Read the model definition and answer for the solid it produces. Units are mm, in the model's axes. Face numbers are marked on the shaded views. A direction names the side the tool comes from. Coordinates: 2 decimals unless noted, no trailing zeros. Write each loop counter-clockwise with the first axis right and the second up, starting at its lowest first coordinate (ties: lowest second). Pieces come first, ordered by that corner, then holes.
Item 1: A tool of negligible diameter and unlimited length cuts with its end or side. For the marked faces 1, 2, 3, 4 and 5, from which of +Z, -Z, +X, -X, +Y, -Y can it reach the whole face along a straight path? Write none if from no direction.
Item 2: This flat-tipped pin is pushed along its axis until it touches: P1, Ø3, axis at x = 24.5, y = 3, coming from the +Z side. Where does it stop, or does it pass through?
Item 3: Straight lines are drawn through the part: probe 1 along X at (y, z) = (1.2, -5); probe 2 along Z at (x, y) = (7, 4.35); probe 3 along X at (y, z) = (3.15, -24). For each, find the intervals that lie inside material, in ascending order.
Item 4: Section A-A (x = 43) is taken. Give the vertices of the cut face in (y, z).
Item 5: Determine the mould class of the marked faces 6, 7, 8 and 9 for opening direction Z: released by +Z, released by -Z, zero draft, split by the parting line, or undercut.
Item 6: Section C-C (x = 27) is taken. Give the vertices of the cut face in (y, z).
Item 7: Section B-B (y = 5.1) is taken. Give the vertices of the cut face in (x, z).
Item 8: Section D-D (z = -24) is taken. Give the vertices of the cut face in (x, y).
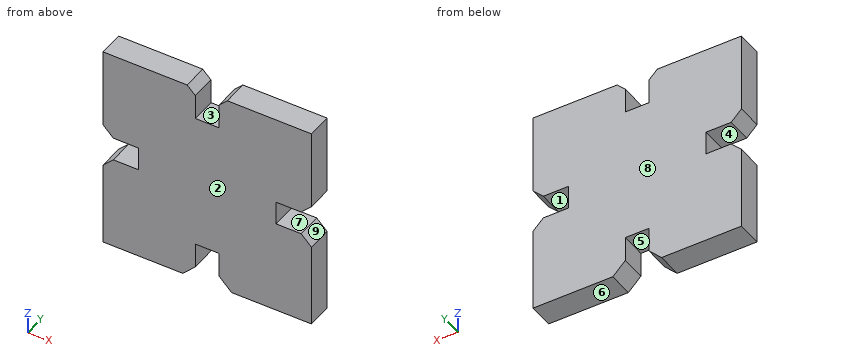
from build123d import *

# Parameters (mm, degrees)
SKETCH1_W           = 50
SKETCH1_H           = 50
BOSS_EXTRUDE1_DEPTH = 6
SKETCH2_W           = 5.7
SKETCH2_H           = 9
CUT_EXTRUDE1_DEPTH  = 6
CHAMFER2_SIZE       = 3
CIRPATTERN4_DEPTH   = 6


# Read off the part's stored shape, not the designer's step: CirPattern4
with BuildPart() as part:
    # Sketch1 → Boss-Extrude1 (new body)
    with BuildSketch(Plane(origin=(0, 0, 0), x_dir=(1, 0, 0), z_dir=(0, 1, 0))):
        with Locations((25, 25)):
            Rectangle(SKETCH1_W, SKETCH1_H)
    extrude(amount=BOSS_EXTRUDE1_DEPTH)

    # Sketch2 → Cut-Extrude1 (cut)
    with BuildSketch(Plane(origin=(0, 6, 0), x_dir=(1, 0, 0), z_dir=(0, 1, 0))):
        with Locations((25, 45.5)):
            Rectangle(SKETCH2_W, SKETCH2_H)
    extrude(amount=-CUT_EXTRUDE1_DEPTH, mode=Mode.SUBTRACT)

    # Chamfer2
    chamfer2_edges = [part.edges().sort_by_distance(p)[0] for p in [
        (22.15, 3, -50),
        (27.85, 3, -50),
    ]]
    chamfer(chamfer2_edges, length=CHAMFER2_SIZE)

    # CirPattern4 outline → CirPattern4 (cut)
    with BuildSketch(Plane(origin=(0, 0, 0), x_dir=(1, 0, 0), z_dir=(0, 1, 0))):
        Polygon((27.85, 7.960814854), (22.15, 7.960814854), (22.15, 1.960814854), (20.189185146, 0), (29.810814854, 0), (27.85, 1.960814854), align=None)
        Polygon((47.519592573, 21.630407427), (50, 19.15), (50, 29.810814854), (47.519592573, 27.330407427), (41.519592573, 27.330407427), (41.519592573, 21.630407427), align=None)
        Polygon((0, 29.810814854), (0, 19.15), (2.480407427, 21.630407427), (8.480407427, 21.630407427), (8.480407427, 27.330407427), (2.480407427, 27.330407427), align=None)
    extrude(amount=CIRPATTERN4_DEPTH, mode=Mode.SUBTRACT)


solid = part.part
Established:
1. face 1: +X, +Y, -Y
1. face 2: +Z, -Z, +X, -X, -Y
1. face 3: +Z, +Y, -Y
1. face 4: -X, +Y, -Y
1. face 5: -Z, +Y, -Y
2. P1: stops at z = -7.96
3. probe 1: x = 0 to 22.15, 27.85 to 50
3. probe 2: z = -50 to -27.33, -21.63 to 0
3. probe 3: x = 8.48 to 41.52
4. outline: (0, -50) - (6, -50) - (6, -27.33) - (0, -27.33) - close; (0, -21.63) - (6, -21.63) - (6, 0) - (0, 0) - close
5. face 6: released by -Z
5. face 7: undercut
5. face 8: zero draft
5. face 9: undercut
6. outline: (0, -41) - (6, -41) - (6, -7.96) - (0, -7.96) - close
7. outline: (0, -50) - (19.15, -50) - (22.15, -47) - (22.15, -41) - (27.85, -41) - (27.85, -47) - (30.85, -50) - (50, -50) - (50, -29.81) - (47.52, -27.33) - (41.52, -27.33) - (41.52, -21.63) - (47.52, -21.63) - (50, -19.15) - (50, 0) - (29.81, 0) - (27.85, -1.96) - (27.85, -7.96) - (22.15, -7.96) - (22.15, -1.96) - (20.19, 0) - (0, 0) - (0, -19.15) - (2.48, -21.63) - (8.48, -21.63) - (8.48, -27.33) - (2.48, -27.33) - (0, -29.81) - close
8. outline: (8.48, 0) - (41.52, 0) - (41.52, 6) - (8.48, 6) - close
